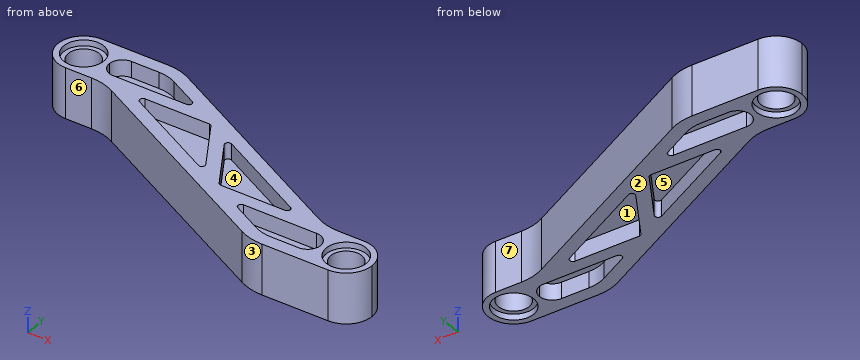
from build123d import *

# Parameters (mm, degrees)
F1_DEPTH  = 3.9
F3_DEPTH  = 2.5
F5_DEPTH  = 2.5
F6_R      = 8
F7_R      = 3.99999
F8_R      = 2.4
F9_DEPTH  = 3.901
F8_R_2    = 3.1
F10_DEPTH = 0.9
F12_R     = 1.99999
F13_R     = 6
F14_R     = 0.5


# Not quite as in the source:
# - a fillet or chamfer is up to 0.001 mm smaller than in the source, because OpenCascade refuses the exact size


with BuildPart() as f1:
    # F0 (on Top) → F1 (new body)
    with BuildSketch(Plane.XY):
        Polygon((-10.2351482974, 8), (-26.5155562797, 8), (-26.5155562797, 0), (-16.5155562797, 0), (19.0857153862, -18.6285724837), (35.3661233686, -18.6285724837), (35.3661233686, -10.6285724837), (25.3661233686, -10.6285724837), align=None)
    extrude(amount=F1_DEPTH)

    # F2 (on face) → F3 (cut)
    with BuildSketch(Plane.XY.offset(3.9)):
        Polygon((24.8744862124, -12.6285724837), (-10.7267854535, 6), (-18.5155562797, 6), (-18.5155562797, 2), (-16.0239191236, 2), (19.5773525424, -16.6285724837), (27.3661233686, -16.6285724837), (27.3661233686, -12.6285724837), align=None)
    extrude(amount=-F3_DEPTH, mode=Mode.SUBTRACT)

    # F4 (on face) → F5 (join, through all)
    with BuildSketch(Plane.XY.offset(3.9)):
        Polygon((11.9329081391, -12.6285724837), (24.8744862124, -12.6285724837), (21.0522640108, -10.6285724837), (8.7555263004, -10.6285724837), (3.1855427267, -1.2797066451), (0.7398811514, 0), (0.0950407885, 0), (5.6650243622, -9.3488658386), align=None)
        Polygon((-12.201696922, 0), (0.0950407885, 0), (-0.1970488953, 0.4902540968), (-3.0823410503, 2), (-16.0239191236, 2), align=None)
        Polygon((-0.1970488953, 0.4902540968), (0.0950407885, 0), (0.7398811514, 0), align=None)
    extrude(amount=-F5_DEPTH)

    # F6
    f6_edges = [f1.edges().sort_by_distance(p)[0] for p in [
        (-10.235148, 8, 1.95),
        (25.366123, -10.628572, 1.95),
        (19.085715, -18.628572, 1.95),
        (-16.515556, 0, 1.95),
    ]]
    fillet(f6_edges, radius=F6_R)

    # F7 (radius 4 in the source; OpenCascade refuses exactly that, so slightly less here)
    f7_edges = [f1.edges().sort_by_distance(p)[0] for p in [
        (-26.515556, 8, 1.95),
        (-26.515556, 0, 1.95),
        (35.366123, -10.628572, 1.95),
        (35.366123, -18.628572, 1.95),
    ]]
    fillet(f7_edges, radius=F7_R)

    # F8 (on face) → F9 (cut, through all)
    with BuildSketch(Plane.XY.offset(3.9)):
        with Locations((-22.5155562797, 4)):
            Circle(F8_R)
        with Locations((31.3661233686, -14.6285724837)):
            Circle(F8_R)
    extrude(amount=-F9_DEPTH, mode=Mode.SUBTRACT)

    # F8 (on face) → F10 (cut)
    with BuildSketch(Plane.XY.offset(3.9)):
        with Locations((-22.5155562797, 4)):
            Circle(F8_R_2)
        with Locations((-22.5155562797, 4)):
            Circle(F8_R, mode=Mode.SUBTRACT)
        with Locations((31.3661233686, -14.6285724837)):
            Circle(F8_R_2)
        with Locations((31.3661233686, -14.6285724837)):
            Circle(F8_R, mode=Mode.SUBTRACT)
    extrude(amount=-F10_DEPTH, mode=Mode.SUBTRACT)

    # F11: F1 across face


with BuildPart() as f1_1:
    add(f1.part)
    add(f1.part.mirror(Plane(origin=(4.4252835444, -5.3142862419, 0), x_dir=(1, 0, 0), z_dir=(0, 0, -1))))

    # F12 (radius 2 in the source; OpenCascade refuses exactly that, so slightly less here)
    f12_edges = [f1_1.edges().sort_by_distance(p)[0] for p in [
        (27.366123, -16.628572, 2.65),
        (27.366123, -12.628572, 2.65),
        (-18.515556, 2, 2.65),
        (-18.515556, 6, 2.65),
        (-18.515556, 2, -2.65),
        (-18.515556, 6, -2.65),
        (27.366123, -16.628572, -2.65),
        (27.366123, -12.628572, -2.65),
    ]]
    fillet(f12_edges, radius=F12_R)

    # F13
    f13_edges = [f1_1.edges().sort_by_distance(p)[0] for p in [
        (19.577353, -16.628572, -2.65),
        (-10.726785, 6, -2.65),
        (-10.726785, 6, 2.65),
        (19.577353, -16.628572, 2.65),
    ]]
    fillet(f13_edges, radius=F13_R)

    # F14
    f14_edges = [f1_1.edges().sort_by_distance(p)[0] for p in [
        (8.755526, -10.628572, 2.65),
        (21.052264, -10.628572, 2.65),
        (3.185543, -1.279707, 2.65),
        (11.932908, -12.628572, 2.65),
        (-12.201697, 0, 2.65),
        (0.095041, 0, 2.65),
        (5.665024, -9.348866, 2.65),
        (-3.082341, 2, 2.65),
        (-3.082341, 2, -2.65),
        (21.052264, -10.628572, -2.65),
        (-12.201697, 0, -2.65),
        (11.932908, -12.628572, -2.65),
        (8.755526, -10.628572, -2.65),
        (3.185543, -1.279707, -2.65),
        (0.095041, 0, -2.65),
        (5.665024, -9.348866, -2.65),
    ]]
    fillet(f14_edges, radius=F14_R)


solid = f1_1.part
Here's how the part is built. I have some questions about the finished solid (model axes, mm). Face numbers are marked on the shaded views. A direction names the side the tool comes from. Round coordinates to 2 decimals unless told otherwise and drop trailing zeros. Return JSON: item names as keys, results as strings. Group by question number.
1. If we section it at A-A on z = 0.75: State how many separate pieces and enclosed holes the cut face has, then the cut area to 3 significant figures.
2. Please list where these lines run through material, in increasing order: probe 1 along X at (y, z) = (-2.75, 3.5); probe 2 along Z at (x, y) = (-15, 5); probe 3 along X at (y, z) = (3, -0.5).
3. If we mould it in two halves opening along Y, with no side actions, what happens to the marked faces 1, 2 and 3? For each: pulls with the +Y half, pulls with the -Y half, needs draft (parallel to the pull), parting line crosses it, or undercut.
4. On a 3-axis mill with a long thin cutter (end or side, diameter ignored), from which of +Z, -Z, +X, -X, +Y, -Y can I reach the whole of each face in a straight line? I mean the marked faces 4, 5, 6 and 7. Say none if no direction works.
5. I'm going to push flat-ended pins straight in: pin 1 Ø2.5 at (x, y) = (8.5, -8) entering from +Z; pin 2 Ø1.5 at (y, z) = (3, -1) entering from -X; pin 3 Ø3 at (y, z) = (-9.5, 2.5) entering from -X; pin 4 Ø2 at (y, z) = (-11, 2) entering from -X. Where does each tip first touch, or does it pass through?
Reply:
{
 "1": {"separate pieces": "1", "enclosed holes": "2", "area": "562 mm^2"},
 "2": {"probe 1": "-11.26 to -6.95, 1.73 to 4.06, 6 to 10.31", "probe 2": "-1.4 to 1.4", "probe 3": "-26.39 to -24.7, -20.33 to -0.68"},
 "3": {"face 1": "undercut", "face 2": "needs draft", "face 3": "pulls with the -Y half"},
 "4": {"face 4": "+Z", "face 5": "-Z", "face 6": "+Z, -Z, -X, -Y", "face 7": "+Z, -Z, +X, +Y"},
 "5": {"pin 1": "z = 3.9", "pin 2": "x = -26.51", "pin 3": "x = -1.23", "pin 4": "x = 2.6"}
}
